Job drawing, mm, ordinate dimensions from the low corner. One solid piece. A direction names the side the tool comes from. Give positions to 0.01 mm unless a question says otherwise; leave off trailing zeros. Order: outer loops, then holes, each group sorted by start corner. A loop starts at its lowest first (then second) coordinate and runs counter-clockwise, first axis right, second up.
1. Slice it at D-D on x = 14. List the corners of the cut face in (y, z), and give its area (3 significant figures).
2. Probe line 1 (Y direction, x = 36.5, z = 44.45); line 2 (Y direction, x = 5, z = 44). List the from-to ranges inside material, lowest first.
3. Mould opens along Z. For the marked faces 3, 4 and 5 say: +Z half, -Z half, draft (parallel to the pull), parting line (faces both ways), or undercut.
4. Slice it at A-A on y = 5.5. List the corners of the cut face in (x, z), and give its area (3 significant figures).
5. Drop flat-ended pins along their axis: pin 1 Ø3.5 at (x, y) = (5.5, 36.5) entering from +Z; pin 2 Ø5 at (x, y) = (5.5, 5.5) entering from -Z; pin 3 Ø2.5 at (x, y) = (5.5, 36.5) entering from +Z; pin 4 Ø10 at (x, y) = (32, 15) entering from +Z. Give the stop position or say it passes through.
6. Which spindle directions (+Z, -Z, +X, -X, +Y, -Y) get a long thin tool onto all of the face, cutting with end or side? Do the marked faces 1 and 2. Say none if no direction does.
7. Slice it at C-C on z = 62.5. List the corners of the cut face in (x, y), and give its area (3 significant figures).
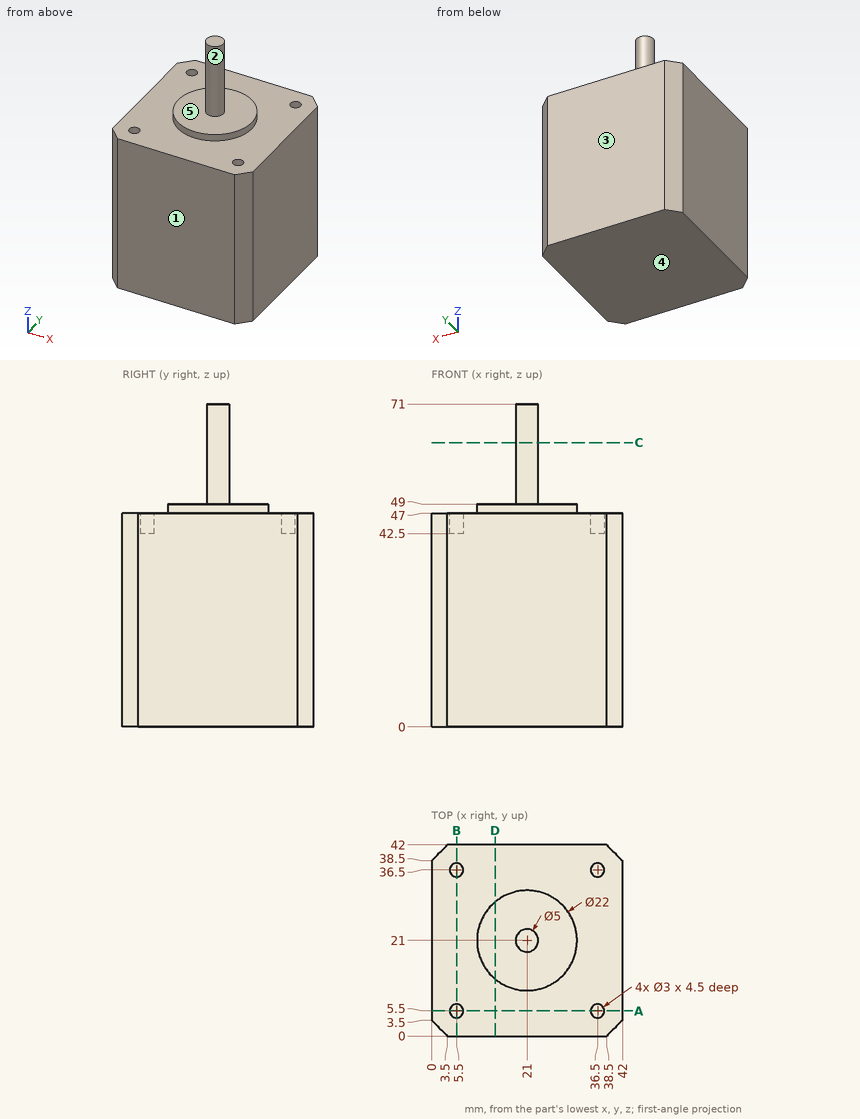
Data:
1. outline: (0, 0) - (42, 0) - (42, 47) - (29.49, 47) - (29.49, 49) - (12.51, 49) - (12.51, 47) - (0, 47) - close
1. area: 2,010 mm2
2. line 1: y = 0 to 4, 7 to 35, 38 to 42
2. line 2: y = 0 to 4.09, 6.91 to 35.09, 37.91 to 42
3. face 3: draft
3. face 4: -Z half
3. face 5: +Z half
4. outline: (0, 0) - (42, 0) - (42, 47) - (38, 47) - (38, 42.5) - (35, 42.5) - (35, 47) - (7, 47) - (7, 42.5) - (4, 42.5) - (4, 47) - (0, 47) - close
4. area: 1,950 mm2
5. pin 1: stops at z = 47
5. pin 2: stops at z = 0
5. pin 3: stops at z = 42.5
5. pin 4: stops at z = 49
6. face 1: +Z, -Z, +X, -X, -Y
6. face 2: +Z
7. outline: circle Ø5 at (21, 21)
7. area: 19.6 mm2
